```python
from build123d import *

# Parameters (mm, degrees)
BOSS_EXTRUDE1_DEPTH      = 25
SKETCH4_R                = 2.5
CUT_EXTRUDE1_DEPTH       = 101.40542814
CUT_EXTRUDE2_DEPTH       = 10
CUT_EXTRUDE2_DEPTH_BACK  = 101.40542814
CUT_EXTRUDE3_DEPTH       = 10
SKETCH8_R                = 9
CUT_EXTRUDE5_DEPTH       = 99.393343271
CUT_EXTRUDE6_REACH       = 102.405
SKETCH11_R               = 14
SKETCH11_R_2             = 9
BOSS_EXTRUDE3_DEPTH      = 8
BOSS_EXTRUDE3_DEPTH_BACK = 14
SKETCH9_R                = 10.595859712
BOSS_EXTRUDE4_DEPTH      = 8
BOSS_EXTRUDE4_DEPTH_BACK = 14
SKETCH12_R               = 2.5
CUT_EXTRUDE7_DEPTH       = 89.217061842
SKETCH13_W               = 193.888130969
SKETCH13_H               = 72.528835421
CUT_EXTRUDE8_DEPTH       = 2
SKETCH14_W               = 198.779610567
SKETCH14_H               = 62.99888379
CUT_EXTRUDE9_DEPTH       = 2
SKETCH15_W               = 31.372938112
SKETCH15_H               = 40
BOSS_EXTRUDE6_DEPTH      = 22
SKETCH16_W               = 77.912477191
SKETCH16_H               = 40.233640204
BOSS_EXTRUDE7_DEPTH      = 10
SKETCH17_R               = 9
CUT_EXTRUDE10_DEPTH      = 10
SKETCH18_R               = 2.25
CUT_EXTRUDE11_DEPTH      = 10
CUT_EXTRUDE12_DEPTH      = 14
CUT_EXTRUDE13_DEPTH      = 14
SKETCH21_R               = 9
SKETCH21_R_2             = 4.5
BOSS_EXTRUDE9_DEPTH      = 3


with BuildPart() as part:
    # Sketch1 → Boss-Extrude1 (new body)
    with BuildSketch(Plane(origin=(0, 0, 0), x_dir=(1, 0, 0), z_dir=(0, 1, 0))):
        with BuildLine():
            Line((-62.5, 30), (62.5, 30))
            ThreePointArc((62.5, 30), (92.5, 0), (62.5, -30))
            Line((62.5, -30), (-62.5, -30))
            ThreePointArc((-62.5, -30), (-92.5, 0), (-62.5, 30))
        make_face()
    extrude(amount=BOSS_EXTRUDE1_DEPTH)

    # Sketch4 → Cut-Extrude1 (cut, through all)
    with BuildSketch(Plane(origin=(0, 25, 0), x_dir=(1, 0, 0), z_dir=(0, 1, 0))):
        with Locations(Location((-62.5, 0, 0), (0, 0, 270))):
            Circle(SKETCH4_R)
    extrude(amount=-CUT_EXTRUDE1_DEPTH, mode=Mode.SUBTRACT)

    # Sketch1_3 → Cut-Extrude2 (cut, two sides)
    with BuildSketch(Plane(origin=(0, 0, 0), x_dir=(1, 0, 0), z_dir=(0, 1, 0))) as cut_extrude2_sk:
        with BuildLine():
            Line((-62.5, 15), (62.5, 15))
            ThreePointArc((62.5, 15), (77.5, 0), (62.5, -15))
            Line((62.5, -15), (-62.5, -15))
            ThreePointArc((-62.5, -15), (-77.5, 0), (-62.5, 15))
        make_face()
    extrude(amount=CUT_EXTRUDE2_DEPTH, mode=Mode.SUBTRACT)
    extrude(cut_extrude2_sk.sketch, amount=-CUT_EXTRUDE2_DEPTH_BACK, mode=Mode.SUBTRACT)

    # Sketch7 → Cut-Extrude3 (cut)
    with BuildSketch(Plane(origin=(0, 25, 0), x_dir=(1, 0, 0), z_dir=(0, 1, 0))):
        with BuildLine():
            Line((-62.5, 15), (62.5, 15))
            ThreePointArc((62.5, 15), (77.5, 0), (62.5, -15))
            Line((62.5, -15), (-62.5, -15))
            ThreePointArc((-62.5, -15), (-77.5, 0), (-62.5, 15))
        make_face()
    extrude(amount=-CUT_EXTRUDE3_DEPTH, mode=Mode.SUBTRACT)

    # Sketch8 → Cut-Extrude5 (cut, through all)
    with BuildSketch(Plane(origin=(0, 10, 0), x_dir=(-1, 0, 0), z_dir=(0, -1, 0))):
        with Locations(Location((-62.5, 0, 0), (0, 0, 90))):
            Circle(SKETCH8_R)
    extrude(amount=-CUT_EXTRUDE5_DEPTH, mode=Mode.SUBTRACT)

    # Sketch10 → Cut-Extrude6 (cut, up to next)
    with BuildSketch(Plane(origin=(0, 25, 0), x_dir=(1, 0, 0), z_dir=(0, 1, 0)), mode=Mode.PRIVATE) as cut_extrude6_sk1:
        with BuildLine():
            Line((-62.5, -30), (62.5, -30))
            ThreePointArc((62.5, -30), (92.5, 0), (62.5, 30))
            Line((62.5, 30), (-62.5, 30))
            ThreePointArc((-62.5, 30), (-92.5, 0), (-62.5, -30))
        make_face()
        with BuildLine():
            Line((-62.5, 20), (62.5, 20))
            ThreePointArc((62.5, 20), (82.5, 0), (62.5, -20))
            Line((62.5, -20), (-62.5, -20))
            ThreePointArc((-62.5, -20), (-82.5, 0), (-62.5, 20))
        make_face(mode=Mode.SUBTRACT)
    cut_extrude6_tool1 = extrude(cut_extrude6_sk1.sketch, amount=-CUT_EXTRUDE6_REACH, mode=Mode.PRIVATE) & part.part
    add(cut_extrude6_tool1.solids().sort_by_distance((0, 25, 28.055135))[0], mode=Mode.SUBTRACT)

    # Sketch11 → Boss-Extrude3 (add, two sides)
    with BuildSketch(Plane(origin=(0, 15, 0), x_dir=(1, 0, 0), z_dir=(0, 1, 0))) as boss_extrude3_sk:
        with Locations(Location((62.5, 0, 0), (0, 0, 270))):
            Circle(SKETCH11_R)
        with Locations(Location((62.5, 0, 0), (0, 0, 90))):
            Circle(SKETCH11_R_2, mode=Mode.SUBTRACT)
    extrude(amount=BOSS_EXTRUDE3_DEPTH)
    extrude(boss_extrude3_sk.sketch, amount=-BOSS_EXTRUDE3_DEPTH_BACK)

    # Sketch9 → Boss-Extrude4 (add, two sides)
    with BuildSketch(Plane(origin=(0, 15, 0), x_dir=(1, 0, 0), z_dir=(0, 1, 0))) as boss_extrude4_sk:
        with Locations(Location((-62.5, 0, 0), (0, 0, 270))):
            Circle(SKETCH9_R)
    extrude(amount=BOSS_EXTRUDE4_DEPTH)
    extrude(boss_extrude4_sk.sketch, amount=-BOSS_EXTRUDE4_DEPTH_BACK)

    # Sketch12 → Cut-Extrude7 (cut, through all)
    with BuildSketch(Plane.XZ.offset(-1)):
        with Locations(Location((-62.5, 0, 0), (0, 0, 270))):
            Circle(SKETCH12_R)
    extrude(amount=-CUT_EXTRUDE7_DEPTH, mode=Mode.SUBTRACT)

    # Sketch13 → Cut-Extrude8 (cut)
    with BuildSketch(Plane(origin=(0, 25, 0), x_dir=(1, 0, 0), z_dir=(0, 1, 0))):
        with Locations((-4.849311671, -4.672767471)):
            Rectangle(SKETCH13_W, SKETCH13_H)
    extrude(amount=-CUT_EXTRUDE8_DEPTH, mode=Mode.SUBTRACT)

    # Sketch14 → Cut-Extrude9 (cut)
    with BuildSketch(Plane.XZ):
        with Locations((0.126503783, -3.704696323)):
            Rectangle(SKETCH14_W, SKETCH14_H)
    extrude(amount=-CUT_EXTRUDE9_DEPTH, mode=Mode.SUBTRACT)

    # Sketch15 → Boss-Extrude6 (add)
    with BuildSketch(Plane(origin=(0, 15, 0), x_dir=(1, 0, 0), z_dir=(0, 1, 0))):
        with Locations((25.047748977, 0)):
            Rectangle(SKETCH15_W, SKETCH15_H)
    extrude(amount=BOSS_EXTRUDE6_DEPTH)

    # Sketch16 → Boss-Extrude7 (add)
    with BuildSketch(Plane(origin=(0, 37, 0), x_dir=(1, 0, 0), z_dir=(0, 1, 0))):
        with Locations((48.317518517, -0.116820102)):
            Rectangle(SKETCH16_W, SKETCH16_H)
    extrude(amount=BOSS_EXTRUDE7_DEPTH)

    # Sketch17 → Cut-Extrude10 (cut)
    with BuildSketch(Plane.XZ.offset(-37)):
        with Locations(Location((62.5, 0, 0), (0, 0, 270))):
            Circle(SKETCH17_R)
    extrude(amount=-CUT_EXTRUDE10_DEPTH, mode=Mode.SUBTRACT)

    # Sketch18 → Cut-Extrude11 (cut)
    with BuildSketch(Plane(origin=(0, 47, 0), x_dir=(1, 0, 0), z_dir=(0, 1, 0))):
        with Locations(Location((27.4, 5, 0), (0, 0, 270))):
            Circle(SKETCH18_R)
        with Locations(Location((27.4, -5, 0), (0, 0, 270))):
            Circle(SKETCH18_R)
        with Locations(Location((77.9, 5, 0), (0, 0, 270))):
            Circle(SKETCH18_R)
        with Locations(Location((77.9, -5, 0), (0, 0, 270))):
            Circle(SKETCH18_R)
    extrude(amount=-CUT_EXTRUDE11_DEPTH, mode=Mode.SUBTRACT)

    # Sketch19 → Cut-Extrude12 (cut)
    with BuildSketch(Plane(origin=(0, 23, 0), x_dir=(1, 0, 0), z_dir=(0, 1, 0))):
        Polygon((62.5, 0), (9.361279921, 20), (62.5, 20), align=None)
    extrude(amount=CUT_EXTRUDE12_DEPTH, mode=Mode.SUBTRACT)

    # Sketch20 → Cut-Extrude13 (cut)
    with BuildSketch(Plane(origin=(0, 23, 0), x_dir=(1, 0, 0), z_dir=(0, 1, 0))):
        Polygon((62.5, 0), (9.361279921, -20), (62.5, -20.233640204), align=None)
    extrude(amount=CUT_EXTRUDE13_DEPTH, mode=Mode.SUBTRACT)

    # Sketch21 → Boss-Extrude9 (add)
    with BuildSketch(Plane.XZ.offset(-37)):
        with Locations(Location((62.5, 0, 0), (0, 0, 270))):
            Circle(SKETCH21_R)
        with Locations(Location((62.5, 0, 0), (0, 0, 270))):
            Circle(SKETCH21_R_2, mode=Mode.SUBTRACT)
    extrude(amount=-BOSS_EXTRUDE9_DEPTH)


solid = part.part
```
Geometry check sheet. Reference: the model listing, model coordinates, mm. A direction names the side the tool comes from. Give positions to 0.01 mm unless a question says otherwise; leave off trailing zeros. Write each loop counter-clockwise with the first axis right and the second up, starting at its lowest first coordinate (ties: lowest second). Pieces come first, ordered by that corner, then holes.
1) Gauge pin test, flat ends, axial feed: pin 1 (4 mm diameter, centred on x = -18.5, z = -6.5, fed in from +Y); pin 2 (3 mm diameter, centred on y = 22.5, z = 8.5, fed in from -X) (3 decimals); pin 3 (1 mm diameter, centred on y = 14.5, z = -0.5, fed in from -X). Record the tip position at first contact, or that the pin passes through.
2) Section check C-C, the plane x = -9.5. Record the boundary of the cut face in (y, z).
3) Material ranges on L1, parallel to X at y = 6.75, z = 0; L2, parallel to X at y = 11.65, z = 0; L3, parallel to Z at x = 73.5, y = 6, recorded low to high.
4) Section check B-B, the plane z = 0. State how many separate pieces and enclosed holes the cut face has, and give its area (3 significant figures).
5) Access from +Z, -Z, +X, -X, +Y, -Y to the whole of each face (thin tool, end or side, straight path). Record for faces 1 (the cylindrical face through (-51.994, 6.056, -1.379)), 2 (the flat face through (52, 19, 15)), 3 (the flat face through (-62, 23, -3)), 4 (the flat face through (-26, 19, 15)).
6) Section check A-A, the plane y = 44.5. Record the boundary of the cut face in (x, z).
7) Release check for a two-part mould opening along X. For faces 5 (the cylindrical face through (76.38, 18.94, -1.82)), 6 (the cylindrical face through (82.495, 12.647, -0.44)), 7 (the flat face through (57.5, 37, 0.4)) record: pulls with the +X half, pulls with the -X half, needs draft (parallel to the pull), parting line crosses it, or undercut.
Computed:
1. pin 1: stops at y = 15
1. pin 2: stops at x = -81.235
1. pin 3: stops at x = -82.5
2. outline: (2, -20) - (23, -20) - (23, -15) - (15, -15) - (15, 15) - (23, 15) - (23, 20) - (2, 20) - (2, 15) - (10, 15) - (10, -15) - (2, -15) - close
3. L1: x = -82.5 to -77.5, -73.1 to -65, -60 to -51.9, 48.5 to 53.5, 71.5 to 76.5, 77.5 to 82.5
3. L2: x = -82.5 to -65, -60 to 53.5, 71.5 to 82.5
3. L3: z = -16.7 to -10.2, -8.66 to 8.66, 10.2 to 16.7
4. separate pieces: 4
4. enclosed holes: 0
4. area: 2,610 mm2
5. face 1: -Y
5. face 2: none
5. face 3: +Z, -Z, -X, +Y
5. face 4: +Y
6. outline: (9.36, -20) - (87.27, -20) - (87.27, 20.23) - (9.36, 20.23) - close; hole circle Ø4.5 at (27.4, -5); hole circle Ø4.5 at (27.4, 5); hole circle Ø18 at (62.5, 0); hole circle Ø4.5 at (77.9, -5); hole circle Ø4.5 at (77.9, 5)
7. face 5: undercut
7. face 6: pulls with the +X half
7. face 7: needs draft
